```python
from build123d import *

# Parameters (mm, degrees)
SKETCH1_R           = 1.5
SKETCH1_R_2         = 1
SKETCH1_R_3         = 4
BOSS_EXTRUDE1_DEPTH = 4.6


with BuildPart() as part:
    # Sketch1 → Boss-Extrude1 (new body)
    with BuildSketch(Plane(origin=(0, 0, 0), x_dir=(1, 0, 0), z_dir=(0, 1, 0))):
        with BuildLine():
            Line((33.841256749, 14.73946958), (36.132184269, 14.73946958))
            ThreePointArc((36.132184269, 14.73946958), (39.75713684, 16.478313044), (41.09081738, 20.271089593))
            Line((41.09081738, 20.271089593), (41.09081738, 28.286294101))
            ThreePointArc((41.09081738, 28.286294101), (39.602380799, 30.901377208), (36.712338736, 31.739088372))
            ThreePointArc((36.712338736, 31.739088372), (33.680921675, 33.128286782), (32.51969773, 36.254133959))
            Line((32.51969773, 36.254133959), (32.51969773, 46.640032758))
            ThreePointArc((32.51969773, 46.640032758), (33.320707465, 48.524930167), (34.713196388, 50.026738889))
            Line((34.713196388, 50.026738889), (34.713196388, 64.026738889))
            Line((34.713196388, 64.026738889), (40.7852702, 68.285935139))
            ThreePointArc((40.7852702, 68.285935139), (42.40733668, 71.23946958), (40.7852702, 74.193004021))
            Line((40.7852702, 74.193004021), (35.075266798, 78.198229556))
            ThreePointArc((35.075266798, 78.198229556), (26.272366536, 78.780683171), (21.694113287, 71.23946958))
            ThreePointArc((21.694113287, 71.23946958), (23.941923331, 48.851382594), (21.694113287, 26.463295609))
            Line((21.694113287, 26.463295609), (21.694113287, 17.463295609))
            ThreePointArc((21.694113287, 17.463295609), (21.954167675, 15.759997208), (23.342467746, 14.73946958))
            Line((23.342467746, 14.73946958), (33.841256749, 14.73946958))
        make_face()
        with Locations((30.194113287, 71.23946958)):
            Circle(SKETCH1_R, mode=Mode.SUBTRACT)
        with Locations((38.90733668, 71.23946958)):
            Circle(SKETCH1_R_2, mode=Mode.SUBTRACT)
        with Locations((23.566412567, 16.94349474)):
            Circle(SKETCH1_R_2, mode=Mode.SUBTRACT)
        with Locations((36.132184269, 26.716174154)):
            Circle(SKETCH1_R_3, mode=Mode.SUBTRACT)
    extrude(amount=BOSS_EXTRUDE1_DEPTH)


solid = part.part
```
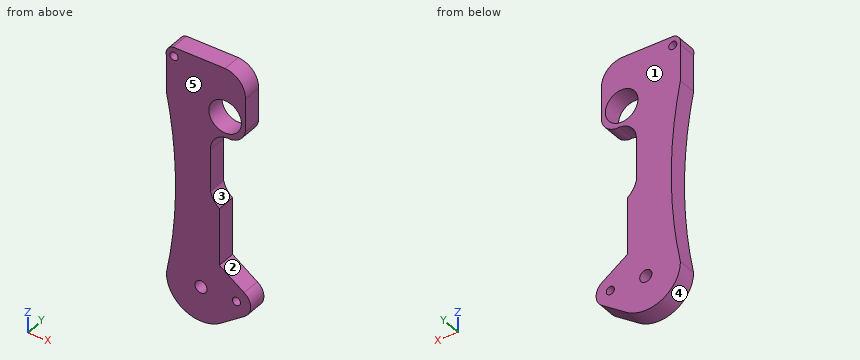
The listing builds one solid part. Answer for the finished solid, in the listing's coordinates (mm). Face numbers are marked on the shaded views. A direction names the side the tool comes from. Round coordinates to 2 decimals unless told otherwise and drop trailing zeros. Loops run counter-clockwise (first coordinate to the right, second up) from the corner with the lowest first, then second, coordinate; pieces in that order, holes last. Notation, with made-up numbers: (-32.75, -25) -> (21.25, -25) arc R19 cw to (21.25, 11) -> close; hole circle Ø6 at (7, -39.5). An arc over 180 degrees is marked (long way). Use one line per item in the form item = value.
1. Flat-ended cylindrical pins translate along their axes: pin 1 Ø2.5 at (y, z) = (2, -22.5) entering from +X; pin 2 Ø2.5 at (y, z) = (3, -21) entering from -X; pin 3 Ø1.4 at (y, z) = (2, -42.5) entering from +X. Find the tip coordinate at first contact, or state that the pin passes through.
Answer key:
pin_1 = 41.09
pin_2 = 21.69
pin_3 = 32.52
2. The part is cut by section C-C on z = -25. Determine the outline of the cut face in (x, y), and give its area (3 significant figures).
Answer key:
outline = (21.69, 0) -> (32.52, 0) -> (32.52, 4.6) -> (21.69, 4.6) -> close; (39.75, 0) -> (41.09, 0) -> (41.09, 4.6) -> (39.75, 4.6) -> close
area = 56.0 mm²
3. The part is cut by section B-B on x = 39. Determine the outline of the cut face in (y, z).
Answer key:
outline = (0, -75.45) -> (4.6, -75.45) -> (4.6, -72.24) -> (0, -72.24) -> close; (0, -70.24) -> (4.6, -70.24) -> (4.6, -67.03) -> (0, -67.03) -> close; (0, -31.29) -> (4.6, -31.29) -> (4.6, -29.5) -> (0, -29.5) -> close; (0, -23.93) -> (4.6, -23.93) -> (4.6, -15.78) -> (0, -15.78) -> close
4. The part is cut by section A-A on x = 31. Determine the outline of the cut face in (y, z).
Answer key:
outline = (0, -79.7) -> (4.6, -79.7) -> (4.6, -72.5) -> (0, -72.5) -> close; (0, -69.97) -> (4.6, -69.97) -> (4.6, -14.74) -> (0, -14.74) -> close
5. A tool of negligible diameter and unlimited length cuts with its end or side. For the marked faces 1 and 2, from which of +Z, -Z, +X, -X, +Y, -Y can it reach the whole face along a straight path? Write none if from no direction.
Answer key:
face_1 = +Z, -Z, +X, -X, +Y
face_2 = +X, +Y, -Y
6. Find the intervals of material crossed by probe 1 along Z at (x, y) = (30, 4.1); probe 2 along Z at (x, y) = (33.5, 1.45); probe 3 along X at (y, z) = (0.45, -26.5), in increasing order. Write a range as [from, to].
Answer key:
probe_1 = [-79.74, -72.73], [-69.75, -14.74]
probe_2 = [-79.07, -48.79], [-33.34, -29.73], [-23.7, -14.74]
probe_3 = [21.7, 32.14], [40.13, 41.09]
7. For a pull along Z with two mould halves and no side action, classify the marked faces 3, 4 and 5 as released by +Z, released by -Z, zero draft, split by the parting line, or undercut.
Answer key:
face_3 = undercut
face_4 = released by -Z
face_5 = zero draft
8. The part is cut by section D-D on y = 1.9. Determine the outline of the cut face in (x, z).
Answer key:
outline = (21.69, -71.24) arc R8.5 ccw to (35.08, -78.2) -> (40.79, -74.19) arc R3.5 ccw to (40.79, -68.29) -> (34.71, -64.03) -> (34.71, -50.03) arc R5.95 cw to (32.52, -46.64) -> (32.52, -36.25) arc R4.36 cw to (36.71, -31.74) arc R4 ccw to (41.09, -28.29) -> (41.09, -20.27) arc R5.25 ccw to (36.13, -14.74) -> (23.34, -14.74) arc R2.25 ccw to (21.69, -17.46) -> (21.69, -26.46) arc R112.62 cw to start; hole circle Ø2 at (23.57, -16.94); hole circle Ø3 at (30.19, -71.24); hole circle Ø8 at (36.13, -26.72); hole circle Ø2 at (38.91, -71.24)
